Source: CAD feature listing. Evaluate the final solid. Frame: model axes, mm. Face numbers are marked on the shaded views. A direction names the side the tool comes from. Coordinates: 2 decimals unless noted, no trailing zeros. Order: outer loops, then holes, each group sorted by start corner. A loop starts at its lowest first (then second) coordinate and runs counter-clockwise, first axis right, second up.
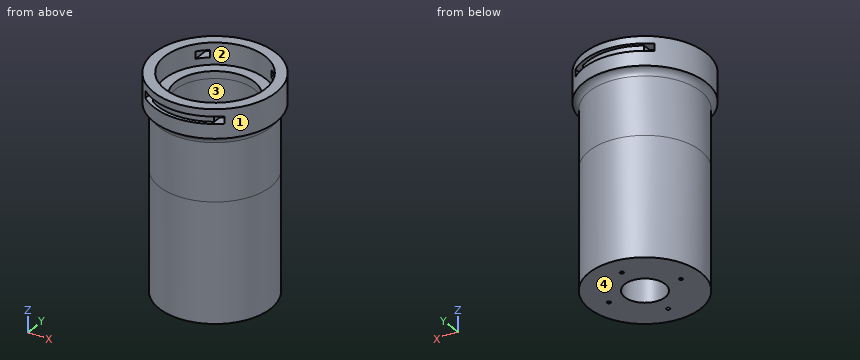
```python
from build123d import *

# Parameters (mm, degrees)
SKETCH1_R                = 15.5
BOSS_EXTRUDE5_DEPTH      = 26
SKETCH3_R                = 5.625
CUT_EXTRUDE2_DEPTH       = 35.007352146
CUT_EXTRUDE3_DEPTH       = 28
CUT_EXTRUDE3_DEPTH_BACK  = 20
SKETCH4_R                = 11.1125
CUT_EXTRUDE6_START       = 6
SKETCH7_R                = 11
SKETCH7_R_2              = 9
CUT_EXTRUDE6_DEPTH       = 2
BOSS_EXTRUDE8_DEPTH      = 6
BOSS_EXTRUDE8_DEPTH_BACK = 2
BOSS_EXTRUDE8_START      = 20
SKETCH12_R               = 17
CUT_EXTRUDE10_START      = 18
SKETCH13_R               = 11
CUT_EXTRUDE10_DEPTH      = 18.411862419
FILLET2_R                = 2
CUT_EXTRUDE11_START      = 26
SKETCH14_R               = 14
CUT_EXTRUDE11_DEPTH      = 6
SKETCH15_R               = 0.5
CUT_EXTRUDE14_DEPTH      = 36.411862419
SKETCH18_W               = 2.5
SKETCH18_H               = 2
CUT_EXTRUDE15_DEPTH      = 20
CUT_EXTRUDE16_DEPTH      = 2
BOSS_EXTRUDE9_START      = 33
SKETCH26_R               = 15.5
SKETCH26_R_2             = 5.625
SKETCH26_R_3             = 0.5
BOSS_EXTRUDE9_DEPTH      = 33


with BuildPart() as part:
    # Sketch1 → Boss-Extrude5 (new body)
    with BuildSketch(Plane.XY):
        Circle(SKETCH1_R)
    extrude(amount=BOSS_EXTRUDE5_DEPTH)

    # Sketch3 → Cut-Extrude2 (cut, through all)
    with BuildSketch(Plane.XY.offset(26)):
        Circle(SKETCH3_R)
    extrude(amount=-CUT_EXTRUDE2_DEPTH, mode=Mode.SUBTRACT)

    # Sketch4 → Cut-Extrude3 (cut, two sides: drawn at the far end of the back side and taken through both)
    with BuildSketch(Plane.XY.offset(26).offset(-CUT_EXTRUDE3_DEPTH_BACK)):
        Circle(SKETCH4_R)
    extrude(amount=CUT_EXTRUDE3_DEPTH + CUT_EXTRUDE3_DEPTH_BACK, mode=Mode.SUBTRACT)

    # Sketch7 → Cut-Extrude6 (cut)
    with BuildSketch(Plane.XY.offset(CUT_EXTRUDE6_START)):
        Circle(SKETCH7_R)
        Circle(SKETCH7_R_2, mode=Mode.SUBTRACT)
    extrude(amount=-CUT_EXTRUDE6_DEPTH, mode=Mode.SUBTRACT)

    # Sketch12 → Boss-Extrude8 (add, two sides: drawn at the far end of the back side and taken through both)
    with BuildSketch(Plane.XY.offset(BOSS_EXTRUDE8_START - BOSS_EXTRUDE8_DEPTH_BACK)):
        Circle(SKETCH12_R)
    extrude(amount=BOSS_EXTRUDE8_DEPTH + BOSS_EXTRUDE8_DEPTH_BACK)

    # Sketch13 → Cut-Extrude10 (cut, through all)
    with BuildSketch(Plane.XY.offset(CUT_EXTRUDE10_START)):
        Circle(SKETCH13_R)
    extrude(amount=CUT_EXTRUDE10_DEPTH, mode=Mode.SUBTRACT)

    # Fillet2
    # the kernel refuses this fillet: 2 mm, written as the material it adds along each edge
    with BuildSketch(Plane(origin=(0, 0, 18), x_dir=(1, 0, 0), z_dir=(0, 1, 0))) as fillet2_piece_1:
        with BuildLine():
            CenterArc((17.5, 1.936491673), FILLET2_R, 180, 75.522487814)
            Line((17, 0), (16.99, -0.038729833))
            ThreePointArc((16.99, -0.038729833), (16.25, -0.04), (15.5, -0.04))
            Line((15.5, -0.04), (15.46, 0))
            Line((15.46, 0), (15.46, 1.936491673))
            Line((15.46, 1.936491673), (15.5, 1.936491673))
        make_face()
    revolve(axis=Axis((0, 0, 18), (0, 0, -1)))

    # Sketch14 → Cut-Extrude11 (cut)
    with BuildSketch(Plane.XY.offset(CUT_EXTRUDE11_START)):
        Circle(SKETCH14_R)
    extrude(amount=-CUT_EXTRUDE11_DEPTH, mode=Mode.SUBTRACT)

    # Sketch15 → Cut-Extrude14 (cut, through all)
    with BuildSketch(Plane.XY):
        with Locations((0, 10)):
            Circle(SKETCH15_R)
        with Locations((0, -10)):
            Circle(SKETCH15_R)
        with Locations((10, 0)):
            Circle(SKETCH15_R)
        with Locations((-10, 0)):
            Circle(SKETCH15_R)
    extrude(amount=CUT_EXTRUDE14_DEPTH, mode=Mode.SUBTRACT)

    # Sketch18 → Cut-Extrude15 (cut, symmetric)
    with BuildSketch(Plane(origin=(0, 0, 0), x_dir=(1, 0, 0), z_dir=(0, 1, 0))):
        with Locations((-9.75, -23)):
            Rectangle(SKETCH18_W, SKETCH18_H)
        with Locations((9.75, -23)):
            Rectangle(SKETCH18_W, SKETCH18_H)
    extrude(amount=CUT_EXTRUDE15_DEPTH, both=True, mode=Mode.SUBTRACT)

    # Sketch23 → Cut-Extrude16 (cut)
    with BuildSketch(Plane(origin=(0, 0, 24), x_dir=(-1, 0, 0), z_dir=(0, 0, -1))):
        with BuildLine():
            Line((9.719197711, 13.947659153), (9.147480199, 13.127208615))
            ThreePointArc((9.147480199, 13.127208615), (0, 16), (-9.147480199, 13.127208615))
            Line((-9.147480199, 13.127208615), (-9.719197711, 13.947659153))
            ThreePointArc((-9.719197711, 13.947659153), (0, 17), (9.719197711, 13.947659153))
        make_face()
        with BuildLine():
            Line((-9.147480199, -13.127208615), (-9.719197711, -13.947659153))
            ThreePointArc((-9.719197711, -13.947659153), (0, -17), (9.719197711, -13.947659153))
            Line((9.719197711, -13.947659153), (9.147480199, -13.127208615))
            ThreePointArc((9.147480199, -13.127208615), (0, -16), (-9.147480199, -13.127208615))
        make_face()
    extrude(amount=CUT_EXTRUDE16_DEPTH, mode=Mode.SUBTRACT)

    # Sketch26 → Boss-Extrude9 (add)
    with BuildSketch(Plane(origin=(0, 0, 0), x_dir=(-1, 0, 0), z_dir=(0, 0, -1)).offset(BOSS_EXTRUDE9_START)):
        Circle(SKETCH26_R)
        with Locations(Location((0, 0, 0), (0, 0, 180))):
            Circle(SKETCH26_R_2, mode=Mode.SUBTRACT)
        with Locations((-10, 0)):
            Circle(SKETCH26_R_3, mode=Mode.SUBTRACT)
        with Locations((0, 10)):
            Circle(SKETCH26_R_3, mode=Mode.SUBTRACT)
        with Locations((10, 0)):
            Circle(SKETCH26_R_3, mode=Mode.SUBTRACT)
        with Locations((0, -10)):
            Circle(SKETCH26_R_3, mode=Mode.SUBTRACT)
    extrude(amount=-BOSS_EXTRUDE9_DEPTH)


solid = part.part
```
Q1. Section query D-D on z = 13. Output: boundary loops of the cut face in (x, y) (1 decimal).
Solutions:
outline: circle Ø31 at (0, 0); hole circle Ø22.2 at (0, 0)
Q2. Section query C-C on y = -12. Give the number of separate pieces and of enclosed holes in the cut face, plus the area to 3 significant figures.
Solutions:
separate pieces: 1
enclosed holes: 2
area: 1,100 mm2
Q3. Material intervals for line 1 along Y through (x, z) = (0, 5) (3 decimals); line 2 along Y through (x, z) = (0, -19.5) (3 decimals); line 3 along Y through (x, z) = (0, 10.5), sorted ascending.
Solutions:
line 1: y = -15.5 to -11, -9 to -5.625, 5.625 to 9, 11 to 15.5
line 2: y = -15.5 to -10.5, -9.5 to -5.625, 5.625 to 9.5, 10.5 to 15.5
line 3: y = -15.5 to -11.11, 11.11 to 15.5
Q4. Pull-direction query (Z, two-part tool) for the marked faces 3 and 4; classes: pulls with the +Z half, pulls with the -Z half, needs draft (parallel to the pull), parting line crosses it, or undercut.
Solutions:
face 3: undercut
face 4: pulls with the -Z half
Q5. Set-up query: the marked faces 1 and 2. Return all of +Z, -Z, +X, -X, +Y, -Y with unobstructed straight access to the full face (end or side cutting, diameter ignored); none if empty.
Solutions:
face 1: +Z, -Z
face 2: +Z
Q6. Section query A-A on z = -13.5. Output: boundary loops of the cut face in (x, y) (3 decimals).
Solutions:
outline: circle Ø31 at (0, 0); hole circle Ø1 at (-10, 0); hole circle Ø11.25 at (0, 0); hole circle Ø1 at (0, -10); hole circle Ø1 at (0, 10); hole circle Ø1 at (10, 0)
Q7. Pin query (flat end, axial travel): P1, Ø1, axis at y = -11.5, z = 23.5, coming from the -X side; P2, Ø1, axis at x = -10.5, z = 1, coming from the +Y side; P3, Ø1.5, axis at y = -6, z = -21, coming from the +X side; P4, Ø10, axis at x = -3, y = 1, coming from the -Z side. Return the tip coordinate at first contact, or that it passes through.
Solutions:
P1: stops at x = -12.96
P2: stops at y = 11.84
P3: stops at x = 14.58
P4: stops at z = -33
Q8. Section query B-B on z = 21. Output: boundary loops of the cut face in (x, y), plus the area to 3 significant figures.
Solutions:
outline: circle Ø34 at (0, 0); hole circle Ø28 at (0, 0)
area: 292 mm2
